from build123d import *

# Parameters (mm, degrees)
SKETCH_1_R          = 1.55
EXTRUDE_1_DEPTH     = 2
FILLET_1_R          = 3
FILLET_2_R          = 1.5
SKETCH_3_R          = 1
CUT_EXTRUDE_1_DEPTH = 5


with BuildPart() as part:
    # 草图1 → 凸台-拉伸1 (new body, symmetric)
    with BuildSketch(Plane.XY):
        Polygon((-10.5, 0), (10.5, 0), (10.5, -7.05), (-1, -7.05), (-1, -10.05), (-6, -10.05), (-10.5, -5.55), align=None)
        with Locations((-7.5, -3)):
            Circle(SKETCH_1_R, mode=Mode.SUBTRACT)
        with Locations((7.5, -3)):
            Circle(SKETCH_1_R, mode=Mode.SUBTRACT)
    extrude(amount=EXTRUDE_1_DEPTH, both=True)

    # 圆角1
    fillet_1_edges = [part.edges().sort_by_distance(p)[0] for p in [
        (-10.5, 0, 0),
        (10.5, 0, 0),
    ]]
    fillet(fillet_1_edges, radius=FILLET_1_R)

    # 圆角2
    fillet_2_edges = [part.edges().sort_by_distance(p)[0] for p in [
        (10.5, -7.05, 0),
        (-6, -10.05, 0),
        (-10.5, -5.55, 0),
    ]]
    fillet(fillet_2_edges, radius=FILLET_2_R)

    # 草图3 → 切除-拉伸1 (cut, through all)
    with BuildSketch(Plane.XY.offset(2)):
        with Locations((0, -7.05)):
            Circle(SKETCH_3_R)
    extrude(amount=-CUT_EXTRUDE_1_DEPTH, mode=Mode.SUBTRACT)


solid = part.part
Could you check a few things on this model? Use its own coordinates, in mm. A direction names the side the tool comes from. Coordinates: 2 decimals unless noted, no trailing zeros. Order: outer loops, then holes, each group sorted by start corner. A loop starts at its lowest first (then second) coordinate and runs counter-clockwise, first axis right, second up. Notation, with made-up numbers: (83.25, -30.5) -> (117.25, -30.5) arc R18 cw to (117.25, 0.5) -> close; hole circle Ø2 at (58, 22.5). An arc over 180 degrees is marked (long way). One line per item, written item: value. Start each with the question number.
1) Imagine slicing it at D-D on y = -6.75. List the corners of the cut face in (x, z) for me, plus the area to 3 significant figures.
2) If I drill on L1, parallel to Y at x = 7.5, z = 0.15; L2, parallel to Y at x = 4, z = -0.6; L3, parallel to Y at x = -7.5, z = -1.6, over which ranges is the centre line in solid material (lowest first)? Write a range as [from, to].
3) Imagine slicing it at B-B on x = -7.25. List the corners of the cut face in (y, z) for me.
4) Imagine slicing it at C-C on y = -4.25. List the corners of the cut face in (x, z) for me, plus the area to 3 significant figures.
5) I'm going to push flat-ended pins straight in: pin 1 (1.2 mm diameter, centred on x = 4, z = -0.5, fed in from -Y); pin 2 (1.9 mm diameter, centred on x = 7.5, y = -3, fed in from -Z). Where does each tip first touch, or does it pass through?
6) Imagine slicing it at A-A on z = 1.25. List the corners of the cut face in (x, y) for me, plus the area to 3 significant figures.
7) Which directions (+Z, -Z, +X, -X, +Y, -Y) give clear straight access to the entire face, cutting with the end or side of a thin tool? Please do faces 1 (the flat face through (5, -7.05, 0)), 2 (the cylindrical face through (-9.6, -0.86, 0.03)).
Answer list:
1. outline: (-9.3, -2) -> (-0.95, -2) -> (-0.95, 2) -> (-9.3, 2) -> close; (0.95, -2) -> (9.9, -2) -> (9.9, 2) -> (0.95, 2) -> close
1. area: 69.2 mm2
2. L1: y = [-7.05, -4.55], [-1.45, 0]
2. L2: y = [-7.05, 0]
2. L3: y = [-8.55, -4.55], [-1.45, 0]
3. outline: (-8.8, -2) -> (-4.53, -2) -> (-4.53, 2) -> (-8.8, 2) -> close; (-1.47, -2) -> (0, -2) -> (0, 2) -> (-1.47, 2) -> close
4. outline: (-10.5, -2) -> (-8.42, -2) -> (-8.42, 2) -> (-10.5, 2) -> close; (-6.58, -2) -> (6.58, -2) -> (6.58, 2) -> (-6.58, 2) -> close; (8.42, -2) -> (10.5, -2) -> (10.5, 2) -> (8.42, 2) -> close
4. area: 69.3 mm2
5. pin 1: stops at y = -7.05
5. pin 2: passes through
6. outline: (-10.5, -4.93) arc R1.5 ccw to (-10.06, -5.99) -> (-6.44, -9.61) arc R1.5 ccw to (-5.38, -10.05) -> (-1, -10.05) -> (-1, -7.05) arc R1 cw to (1, -7.05) -> (9, -7.05) arc R1.5 ccw to (10.5, -5.55) -> (10.5, -3) arc R3 ccw to (7.5, 0) -> (-7.5, 0) arc R3 ccw to (-10.5, -3) -> close; hole circle Ø3.1 at (-7.5, -3); hole circle Ø3.1 at (7.5, -3)
6. area: 145 mm2
7. face 1: +Z, -Z, +X, -Y
7. face 2: +Z, -Z, -X, +Y
